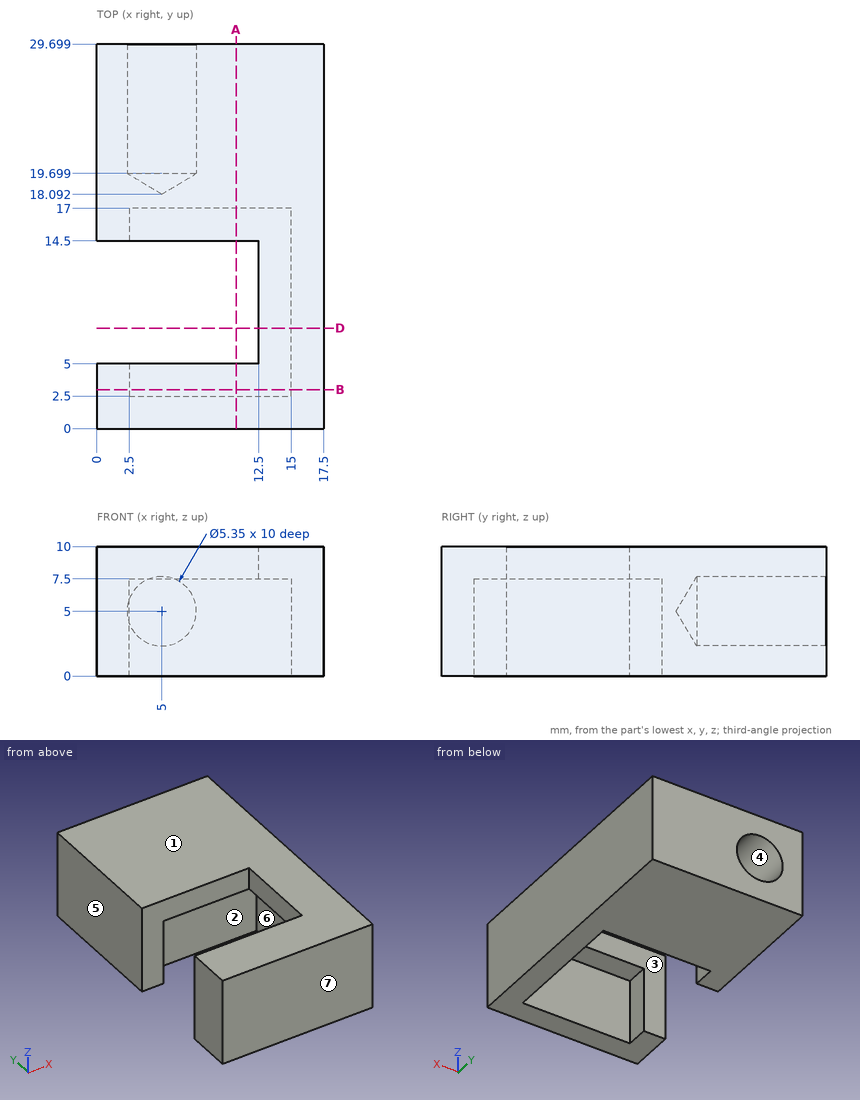
Drawing for the job (mm, zero at the part's lowest x, y, z). A direction names the side the tool comes from. Round coordinates to 2 decimals unless told otherwise and drop trailing zeros. Write each loop counter-clockwise with the first axis right and the second up, starting at its lowest first coordinate (ties: lowest second). Pieces come first, ordered by that corner, then holes. Notation, with made-up numbers: M 24,25 L 29,25 A11 cw 29,46 Z; hole C -5.75,23.25 d10. An arc over 180 degrees is marked long. Answer in a Markdown table with one row per item.
1. Flat gauge pins, fed straight in: P1, Ø2, axis at y = 10.5, z = 8.5, coming from the -X side; P2, Ø6, axis at x = 8, y = 8.5, coming from the -Z side. Where does each tip first touch, or does it go through?
Geometry check:
| item | result |
|---|---|
| P1 | x = 12.5 |
| P2 | through |
2. Saw through at B-B (y = 3). List the corners of the cut face in (x, z).
Geometry check:
| item | result |
|---|---|
| outline | M 0,0 L 2.5,0 L 2.5,7.5 L 15,7.5 L 15,0 L 17.5,0 L 17.5,10 L 0,10 Z |
3. Saw through at D-D (y = 7.75). List the corners of the cut face in (x, z).
Geometry check:
| item | result |
|---|---|
| outline | M 12.5,7.5 L 15,7.5 L 15,0 L 17.5,0 L 17.5,10 L 12.5,10 Z |
4. Probe L1, parallel to X at y = 27, z = 5 (1 decimal); L2, parallel to Z at x = 5, y = 24 (1 decimal); L3, parallel to Y at x = 11, z = 1.5. List the from-to ranges inside material, lowest first. Write a range as [from, to].
Geometry check:
| item | result |
|---|---|
| L1 | [0, 2.3], [7.7, 17.5] |
| L2 | [0, 2.3], [7.7, 10] |
| L3 | [0, 2.5], [17, 29.7] |
5. Mould opens along X. For the marked faces 4, 5, 6 and 7 say: +X half, -X half, draft (parallel to the pull), parting line (faces both ways), or undercut.
Geometry check:
| item | result |
|---|---|
| face 4 | undercut |
| face 5 | -X half |
| face 6 | undercut |
| face 7 | draft |
6. Saw through at A-A (x = 10.75). List the corners of the cut face in (y, z).
Geometry check:
| item | result |
|---|---|
| outline | M 0,0 L 2.5,0 L 2.5,7.5 L 5,7.5 L 5,10 L 0,10 Z; M 14.5,7.5 L 17,7.5 L 17,0 L 29.7,0 L 29.7,10 L 14.5,10 Z |
7. Which spindle directions (+Z, -Z, +X, -X, +Y, -Y) get a long thin tool onto all of the face, cutting with end or side? Do the marked faces 1, 2 and 3. Say none if no direction does.
Geometry check:
| item | result |
|---|---|
| face 1 | +Z, +X, -X, +Y, -Y |
| face 2 | -Z |
| face 3 | +Z, -Z, -X |
